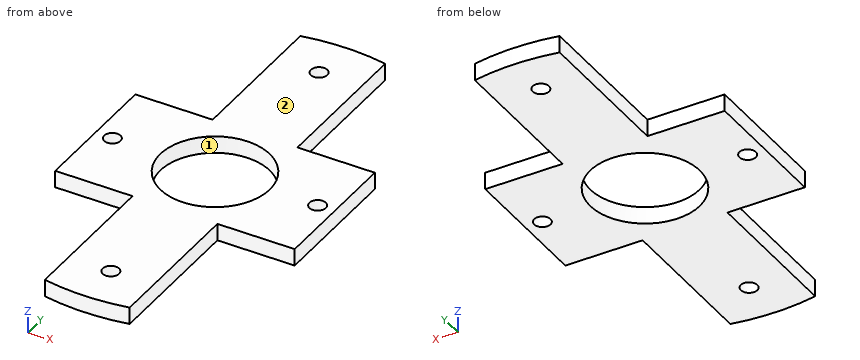
from build123d import *

# Parameters (mm, degrees)
SKETCH1_R           = 15.99
SKETCH1_R_2         = 2.4
BOSS_EXTRUDE1_DEPTH = 5


with BuildPart() as part:
    # Sketch1 → Boss-Extrude1 (new body)
    with BuildSketch(Plane.XY):
        with BuildLine():
            Line((12.4, 20), (35, 20))
            Line((35, 20), (35, 0))
            Line((35, 0), (35, -20))
            Line((35, -20), (12.4, -20))
            Line((12.4, -20), (12.4, -63.806269284))
            ThreePointArc((12.4, -63.806269284), (0, -65), (-12.4, -63.806269284))
            Line((-12.4, -63.806269284), (-12.4, -20))
            Line((-12.4, -20), (-35, -20))
            Line((-35, -20), (-35, 20))
            Line((-35, 20), (-12.4, 20))
            Line((-12.4, 20), (-12.4, 63.806269284))
            ThreePointArc((-12.4, 63.806269284), (0, 65), (12.4, 63.806269284))
            Line((12.4, 63.806269284), (12.4, 20))
        make_face()
        Circle(SKETCH1_R, mode=Mode.SUBTRACT)
        with Locations((0, 52)):
            Circle(SKETCH1_R_2, mode=Mode.SUBTRACT)
        with Locations((30, 0)):
            Circle(SKETCH1_R_2, mode=Mode.SUBTRACT)
        with Locations(Location((0, -52, 0), (0, 0, 180))):
            Circle(SKETCH1_R_2, mode=Mode.SUBTRACT)
        with Locations(Location((-30, 0, 0), (0, 0, 180))):
            Circle(SKETCH1_R_2, mode=Mode.SUBTRACT)
    extrude(amount=BOSS_EXTRUDE1_DEPTH)


solid = part.part
The listing builds one solid part. Answer for the finished solid, in the listing's coordinates (mm). Face numbers are marked on the shaded views. Coordinates: 2 decimals unless noted, no trailing zeros. Order: outer loops, then holes, each group sorted by start corner. A loop starts at its lowest first (then second) coordinate and runs counter-clockwise, first axis right, second up.
Q1. A cutting plane is placed at B-B, the plane y = 52. Write down the section's boundary in (x, z).
Q2. Consider line 1 (Y direction, x = 0, z = 1.5); line 2 (Y direction, x = 30, z = 2.2); line 3 (X direction, y = 1.5, z = 3.05). Determine where each line is inside the solid, lowest interval first.
Q3. A cutting plane is placed at A-A, the plane x = 0. Write down the section's boundary in (y, z).
Q4. A cutting plane is placed at C-C, the plane x = 30. Write down the section's boundary in (y, z), and give its area (3 significant figures).
Q5. A cutting plane is placed at D-D, the plane z = 0.95. Write down the section's boundary in (x, y), and give its area (3 significant figures).
Q6. For a pull along Y with two mould halves and no side action, classify the marked faces 1 and 2 as pulls with the +Y half, pulls with the -Y half, needs draft (parallel to the pull), parting line crosses it, or undercut.
Q7. Given P1, Ø1, axis at x = 9, z = 2.5, coming from the +Y side; P2, Ø1.5, axis at y = -35, z = 2, coming from the +X side; P3, Ø3, axis at x = -20.5, z = 2.5, coming from the -Y side; P4, Ø3, axis at x = -30, y = 0, coming from the -Z side, each flat-ended and moving along its own axis, determine where each tip first touches the part or whether it passes through.
Answers follow:
1. outline: (-12.4, 0) - (-2.4, 0) - (-2.4, 5) - (-12.4, 5) - close; (2.4, 0) - (12.4, 0) - (12.4, 5) - (2.4, 5) - close
2. line 1: y = -65 to -54.4, -49.6 to -15.99, 15.99 to 49.6, 54.4 to 65
2. line 2: y = -20 to -2.4, 2.4 to 20
2. line 3: x = -35 to -31.87, -28.13 to -15.92, 15.92 to 28.13, 31.87 to 35
3. outline: (-65, 0) - (-54.4, 0) - (-54.4, 5) - (-65, 5) - close; (-49.6, 0) - (-15.99, 0) - (-15.99, 5) - (-49.6, 5) - close; (15.99, 0) - (49.6, 0) - (49.6, 5) - (15.99, 5) - close; (54.4, 0) - (65, 0) - (65, 5) - (54.4, 5) - close
4. outline: (-20, 0) - (-2.4, 0) - (-2.4, 5) - (-20, 5) - close; (2.4, 0) - (20, 0) - (20, 5) - (2.4, 5) - close
4. area: 176 mm2
5. outline: (-35, -20) - (-12.4, -20) - (-12.4, -63.81) arc R65 ccw to (12.4, -63.81) - (12.4, -20) - (35, -20) - (35, 20) - (12.4, 20) - (12.4, 63.81) arc R65 ccw to (-12.4, 63.81) - (-12.4, 20) - (-35, 20) - close; hole circle Ø4.8 at (-30, 0); hole circle Ø31.98 at (0, 0); hole circle Ø4.8 at (0, -52); hole circle Ø4.8 at (0, 52); hole circle Ø4.8 at (30, 0)
5. area: 4,140 mm2
6. face 1: undercut
6. face 2: needs draft
7. P1: stops at y = 64.44
7. P2: stops at x = 12.4
7. P3: stops at y = -20
7. P4: passes through
